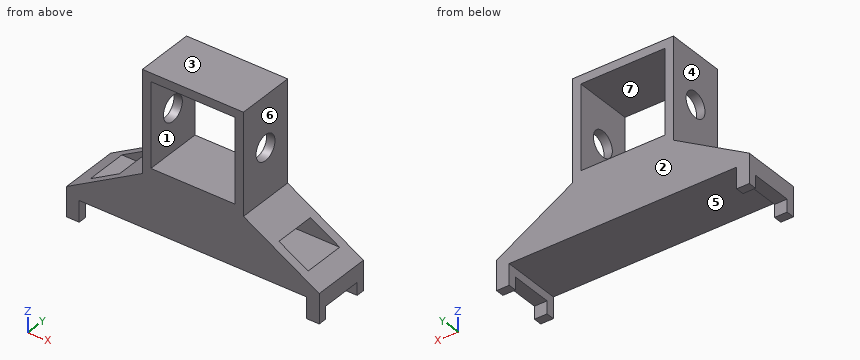
from build123d import *

# Parameters (mm, degrees)
SKETCH_1_W          = 12
SKETCH_1_H          = 12
EXTRUDE_1_DEPTH     = 7
SKETCH_2_W          = 10
SKETCH_2_H          = 10
CUT_EXTRUDE_1_DEPTH = 8
SKETCH_4_R          = 1.5
CUT_EXTRUDE_2_DEPTH = 22
SKETCH_5_W          = 27
SKETCH_5_H          = 2.5
CUT_EXTRUDE_3_DEPTH = 8
SKETCH_6_W          = 2
SKETCH_6_H          = 5
CUT_EXTRUDE_4_DEPTH = 31
SKETCH_7_W          = 1.5
SKETCH_7_H          = 5
CUT_EXTRUDE_5_DEPTH = 31


with BuildPart() as part:
    # Эскиз1 → Бобышка-Вытянуть1 (new body)
    with BuildSketch(Plane(origin=(0, 0, 0), x_dir=(1, 0, 0), z_dir=(0, 1, 0))):
        with Locations((0, 6)):
            Rectangle(SKETCH_1_W, SKETCH_1_H)
        Polygon((-15, 17.196152423), (-6, 12), (6, 12), (15, 17.196152423), (15, 20.696152423), (-15, 20.696152423), align=None)
    extrude(amount=EXTRUDE_1_DEPTH)

    # Эскиз2 → Вырез-Вытянуть1 (cut, through all)
    with BuildSketch(Plane(origin=(0, 7, 0), x_dir=(1, 0, 0), z_dir=(0, 1, 0))):
        with Locations((0, 6)):
            Rectangle(SKETCH_2_W, SKETCH_2_H)
    extrude(amount=-CUT_EXTRUDE_1_DEPTH, mode=Mode.SUBTRACT)

    # Эскиз4 → Вырез-Вытянуть2 (cut, through all)
    with BuildSketch(Plane.ZY.offset(6)):
        with Locations((-6, 3.5)):
            Circle(SKETCH_4_R)
    extrude(amount=-CUT_EXTRUDE_2_DEPTH, mode=Mode.SUBTRACT)

    # Эскиз5 → Вырез-Вытянуть3 (cut, through all)
    with BuildSketch(Plane.XZ):
        with Locations((0, -19.446152423)):
            Rectangle(SKETCH_5_W, SKETCH_5_H)
    extrude(amount=-CUT_EXTRUDE_3_DEPTH, mode=Mode.SUBTRACT)

    # Эскиз6 → Вырез-Вытянуть4 (cut, through all)
    with BuildSketch(Plane(origin=(15, 0, 0), x_dir=(0, 0, -1), z_dir=(1, 0, 0))):
        with Locations((15, 3.5)):
            Rectangle(SKETCH_6_W, SKETCH_6_H)
    extrude(amount=-CUT_EXTRUDE_4_DEPTH, mode=Mode.SUBTRACT)

    # Эскиз7 → Вырез-Вытянуть5 (cut, through all)
    with BuildSketch(Plane.ZY.offset(15)):
        with Locations((-19.946152423, 3.5)):
            Rectangle(SKETCH_7_W, SKETCH_7_H)
    extrude(amount=-CUT_EXTRUDE_5_DEPTH, mode=Mode.SUBTRACT)


solid = part.part
The model under review builds one solid part; all positions refer to its coordinate system, in mm. Face numbers are marked on the shaded views. A direction names the side the tool comes from. Give positions to 0.01 mm unless a question says otherwise; leave off trailing zeros. Loops run counter-clockwise (first coordinate to the right, second up) from the corner with the lowest first, then second, coordinate; pieces in that order, holes last. Notation, with made-up numbers: (-3, -34) -> (42, -34) arc R34 cw to (42, 3) -> close; hole circle Ø7 at (-39.75, 9). An arc over 180 degrees is marked (long way). Answer as a JSON object with one key per item and string values. Group by question number.
Q1. Take a section at B-B (y = 5.5). Write out the cut boundary in (x, z).
Q2. Draft analysis for pull direction Z (two halves, no side actions). For the marked faces 1, 2 and 3, state which applies: pulls with the +Z half, pulls with the -Z half, needs draft (parallel to the pull), parting line crosses it, or undercut.
Q3. Take a section at A-A (x = -1.75). Write out the cut boundary in (y, z).
Q4. Wall thickness on line 1 along Z through (x, y) = (-4.5, 5.5); line 2 along X through (y, z) = (0.5, -4); line 3 along Y through (x, z) = (5.4, -6): over which ranges is each line inside the solid? List them lowest first.
Q5. Take a section at C-C (z = -8.5). Write out the cut boundary in (x, y), plus the area to 3 significant figures.
Q6. Tool access review of the marked faces 4, 5, 6 and 7: name each direction out of +Z, -Z, +X, -X, +Y, -Y from which nothing blocks a thin tool from reaching the whole face with its end or side.
Q7. Take a section at D-D (y = 3.5). Write out the cut boundary in (x, z).
Q8. Insertion check: pin 1 (4 mm diameter, centred on x = 11, y = 3.5, fed in from +Z); pin 2 (2 mm diameter, centred on x = 3, y = 5, fed in from -Z); pin 3 (3 mm diameter, centred on y = 4.5, z = -13, fed in from +X). Each pin has a flat end and moves straight along its axis. Give the tip position at first contact, or say it passes through.
Answer below:
{
 "1": {"outline": "(-15, -19.2) -> (-13.5, -19.2) -> (-13.5, -18.2) -> (13.5, -18.2) -> (13.5, -19.2) -> (15, -19.2) -> (15, -17.2) -> (12.93, -16) -> (-12.93, -16) -> (-15, -17.2) -> close; (-9.46, -14) -> (9.46, -14) -> (6, -12) -> (6, 0) -> (-6, 0) -> (-6, -12) -> close; hole (-5, -11) -> (5, -11) -> (5, -1) -> (-5, -1) -> close"},
 "2": {"face 1": "undercut", "face 2": "needs draft", "face 3": "pulls with the +Z half"},
 "3": {"outline": "(0, -18.2) -> (7, -18.2) -> (7, -11) -> (0, -11) -> close; (0, -1) -> (7, -1) -> (7, 0) -> (0, 0) -> close; hole (1, -16) -> (6, -16) -> (6, -14) -> (1, -14) -> close"},
 "4": {"line 1": "z = -18.2 to -16, -14 to -11, -1 to 0", "line 2": "x = -6 to -5, 5 to 6", "line 3": "y = 0 to 2, 5 to 7"},
 "5": {"outline": "(-6, 0) -> (-5, 0) -> (-5, 7) -> (-6, 7) -> close; (5, 0) -> (6, 0) -> (6, 7) -> (5, 7) -> close", "area": "14.0 mm2"},
 "6": {"face 4": "+Z, -X, +Y, -Y", "face 5": "-Z, +Y, -Y", "face 6": "+Z, +X, +Y, -Y", "face 7": "+Y, -Y"},
 "7": {"outline": "(-15, -19.2) -> (-13.5, -19.2) -> (-13.5, -18.2) -> (13.5, -18.2) -> (13.5, -19.2) -> (15, -19.2) -> (15, -17.2) -> (12.93, -16) -> (-12.93, -16) -> (-15, -17.2) -> close; (-9.46, -14) -> (9.46, -14) -> (6, -12) -> (6, -7.5) -> (5, -7.5) -> (5, -11) -> (-5, -11) -> (-5, -7.5) -> (-6, -7.5) -> (-6, -12) -> close; (-6, -4.5) -> (-5, -4.5) -> (-5, -1) -> (5, -1) -> (5, -4.5) -> (6, -4.5) -> (6, 0) -> (-6, 0) -> close"},
 "8": {"pin 1": "stops at z = -13.73", "pin 2": "stops at z = -18.2", "pin 3": "stops at x = 9.46"}
}
